Can you work these out from the drawing? Everything is in mm from the part's minimum corner. A direction names the side the tool comes from. Give positions to 0.01 mm unless a question says otherwise; leave off trailing zeros. Loops run counter-clockwise (first coordinate to the right, second up) from the corner with the lowest first, then second, coordinate; pieces in that order, holes last. Notation, with made-up numbers: (20.5, -38) -> (60.5, -38) arc R25 ccw to (60.5, -5) -> close; hole circle Ø2 at (67, 8). An arc over 180 degrees is marked (long way). Write item = value, one per line. Start each with the question number.
1) On a 3-axis mill with a long thin cutter (end or side, diameter ignored), from which of +Z, -Z, +X, -X, +Y, -Y can I reach the whole of each face in a straight line? I mean the marked faces 4, 5 and 6. Say none if no direction works.
2) If we mould it in two halves opening along Z, with no side actions, what happens to the marked faces 1, 2 and 3? For each: +Z half, -Z half, draft (parallel to the pull), parting line (faces both ways), or undercut.
3) I want a section at A-A (z = 3). List the corners of the cut face in (x, y) for me, and give its area (3 significant figures).
4) I want a section at B-B (x = 3.25). List the corners of the cut face in (y, z) for me.
5) I want a section at C-C (z = 0.65). List the corners of the cut face in (x, y) for me.
6) I want a section at D-D (y = 10.25). List the corners of the cut face in (x, z) for me.
7) I'm going to push flat-ended pins straight in: pin 1 Ø2 at (x, y) = (9, 3) entering from +Z; pin 2 Ø3 at (y, z) = (4, 1.5) entering from -X; pin 3 Ø1.8 at (y, z) = (3, 2.5) entering from +X. Where does each tip first touch, or does it pass through?
8) I need wall thicknesses on probe 1 along X at (y, z) = (3, 2.8); probe 2 along X at (y, z) = (9.45, 3); probe 3 along Z at (x, y) = (36.75, 10.55). Which ranges of each line are inside material? Lowest first, please. Write a range as from..to.
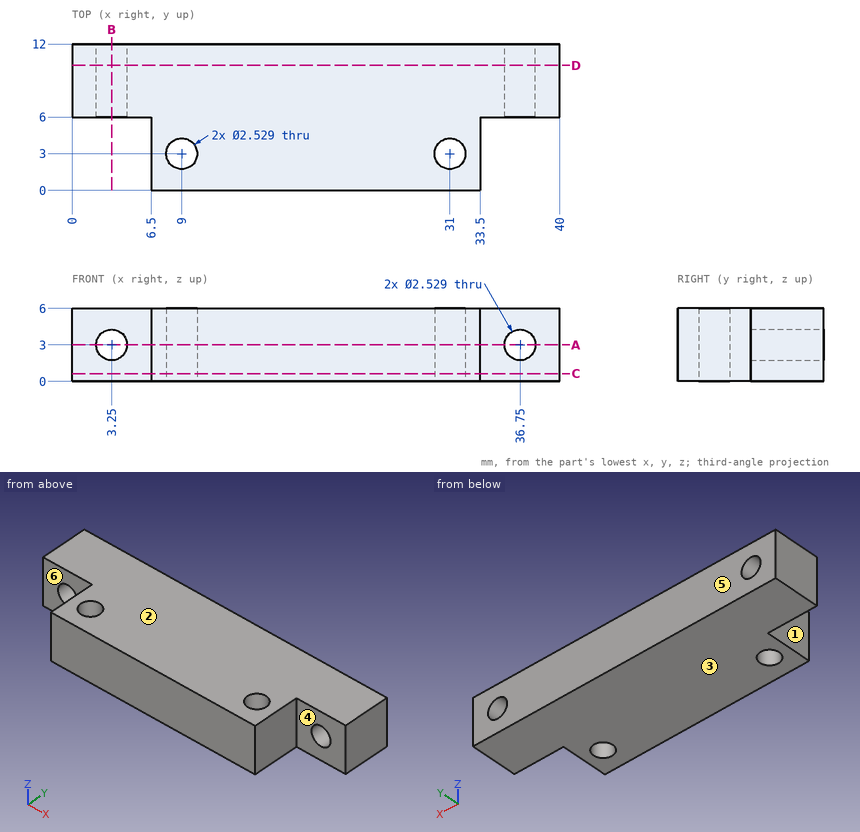
Answer list:
q1.face_4 = +Z, -Z, +X, -Y
q1.face_5 = +Z, -Z, +X, -X, +Y
q1.face_6 = +Z, -Z, -X, -Y
q2.face_1 = draft
q2.face_2 = +Z half
q2.face_3 = -Z half
q3.outline = (0, 6) -> (1.99, 6) -> (1.99, 12) -> (0, 12) -> close; (4.51, 6) -> (6.5, 6) -> (6.5, 0) -> (33.5, 0) -> (33.5, 6) -> (35.49, 6) -> (35.49, 12) -> (4.51, 12) -> close; (38.01, 6) -> (40, 6) -> (40, 12) -> (38.01, 12) -> close; hole circle Ø2.53 at (9, 3); hole circle Ø2.53 at (31, 3)
q3.area = 362 mm^2
q4.outline = (6, 0) -> (12, 0) -> (12, 1.74) -> (6, 1.74) -> close; (6, 4.26) -> (12, 4.26) -> (12, 6) -> (6, 6) -> close
q5.outline = (0, 6) -> (6.5, 6) -> (6.5, 0) -> (33.5, 0) -> (33.5, 6) -> (40, 6) -> (40, 12) -> (0, 12) -> close; hole circle Ø2.53 at (9, 3); hole circle Ø2.53 at (31, 3)
q6.outline = (0, 0) -> (40, 0) -> (40, 6) -> (0, 6) -> close; hole circle Ø2.53 at (3.25, 3); hole circle Ø2.53 at (36.75, 3)
q7.pin_1 = through
q7.pin_2 = 6.5
q7.pin_3 = 33.5
q8.probe_1 = 6.5..7.74, 10.26..29.74, 32.26..33.5
q8.probe_2 = 0..1.99, 4.51..35.49, 38.01..40
q8.probe_3 = 0..1.74, 4.26..6
